For this review, use the dimensioned drawing (mm, ordinates from the lowest corner) and the shaded views. Give positions to 0.01 mm unless a question says otherwise; leave off trailing zeros. Write each loop counter-clockwise with the first axis right and the second up, starting at its lowest first coordinate (ties: lowest second). Pieces come first, ordered by that corner, then holes. Notation, with made-up numbers: (-25.75, 70) -> (-8.75, 70) arc R15 ccw to (-8.75, 86) -> close; hole circle Ø7 at (4.5, -23.5). An arc over 180 degrees is marked (long way). Return JSON: item names as keys, results as strings.
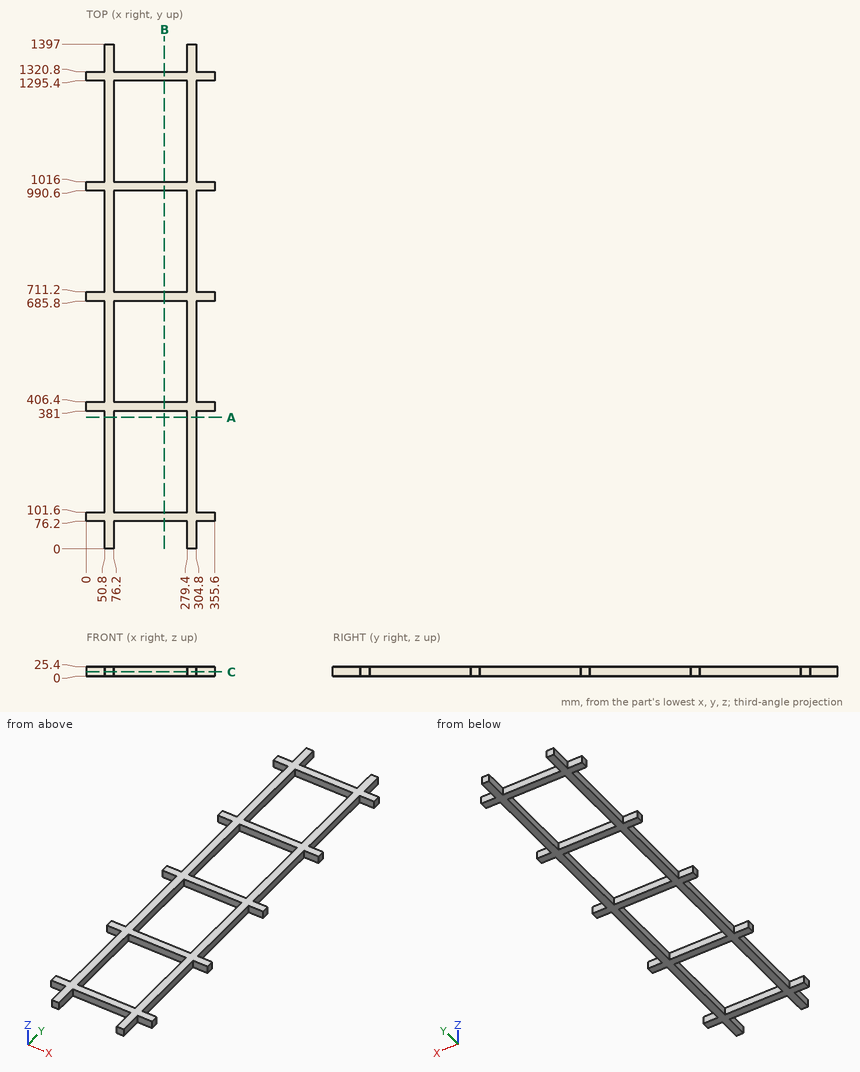
1. Add section C-C, the plane z = 11.5. Count the separate pieces of the cut face and the enclosed holes in it, plus the area to 3 significant figures.
Results found:
{"separate pieces": "1", "enclosed holes": "4", "area": "110,000 mm²"}
2. To check wall thickness, follow probe 1 along Y at (x, z) = (259.5, 18.5); probe 2 along X at (y, z) = (1124, 10.5). State the ranges of each line that lie inside material, in increasing order.
Results found:
{"probe 1": "y = 76.2 to 101.6, 381 to 406.4, 685.8 to 711.2, 990.6 to 1016, 1295.4 to 1320.8", "probe 2": "x = 50.8 to 76.2, 279.4 to 304.8"}
3. Add section B-B, the plane x = 216. State the section outline as (y, z) points.
Results found:
{"outline": "(76.2, 0) -> (101.6, 0) -> (101.6, 25.4) -> (76.2, 25.4) -> close; (381, 0) -> (406.4, 0) -> (406.4, 25.4) -> (381, 25.4) -> close; (685.8, 0) -> (711.2, 0) -> (711.2, 25.4) -> (685.8, 25.4) -> close; (990.6, 0) -> (1016, 0) -> (1016, 25.4) -> (990.6, 25.4) -> close; (1295.4, 0) -> (1320.8, 0) -> (1320.8, 25.4) -> (1295.4, 25.4) -> close"}
4. Add section A-A, the plane y = 364. State the section outline as (x, z) points.
Results found:
{"outline": "(50.8, 0) -> (76.2, 0) -> (76.2, 25.4) -> (50.8, 25.4) -> close; (279.4, 0) -> (304.8, 0) -> (304.8, 25.4) -> (279.4, 25.4) -> close"}
5. For pin 1 (7.5 mm diameter, centred on x = 334, z = 18.5, fed in from +Y); pin 2 (7.5 mm diameter, centred on y = 28.5, z = 17.5, fed in from -X); pin 3 (1.5 mm diameter, centred on x = 154, z = 14, fed in from -Y), all flat-tipped, find the tip position at first contact; note any pin that passes through.
Results found:
{"pin 1": "stops at y = 1320.8", "pin 2": "stops at x = 50.8", "pin 3": "stops at y = 76.2"}
